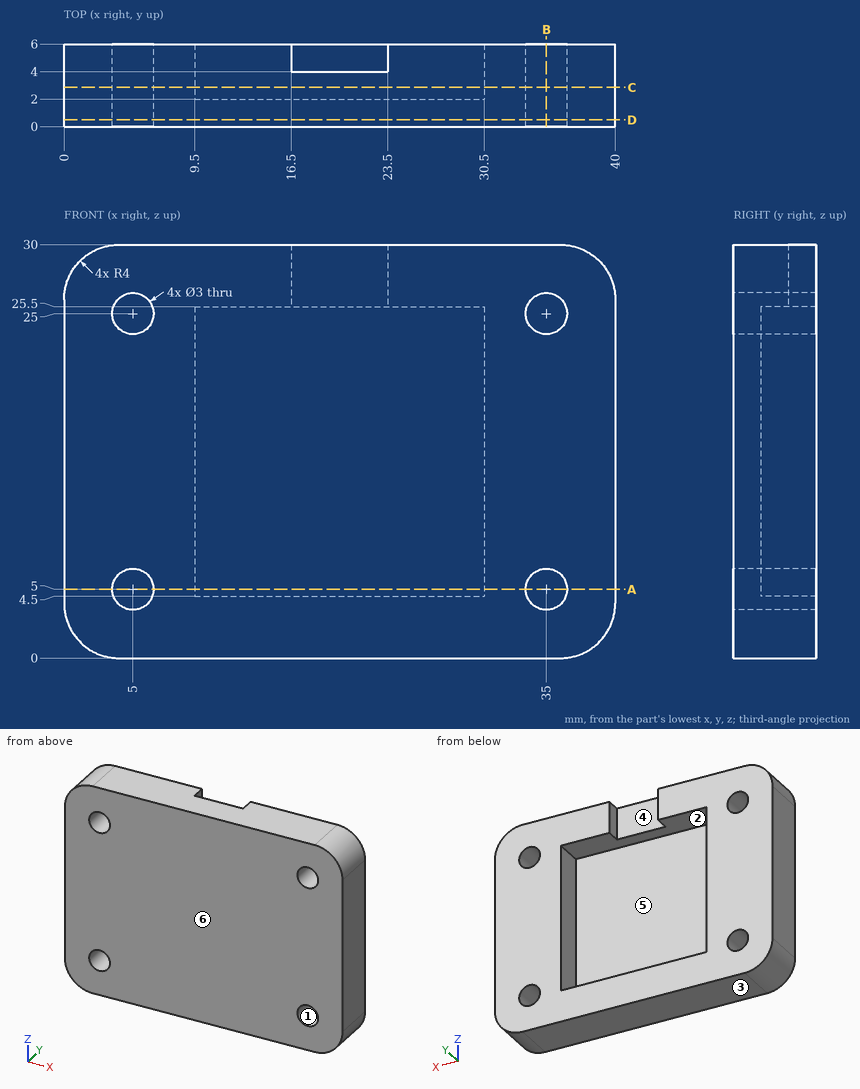
Drawing for the job (mm, zero at the part's lowest x, y, z). A direction names the side the tool comes from. Coordinates: 2 decimals unless noted, no trailing zeros. Loops run counter-clockwise (first coordinate to the right, second up) from the corner with the lowest first, then second, coordinate; pieces in that order, holes last. Notation, with made-up numbers: (68.5, -10) - (115.5, -10) arc R15 ccw to (115.5, 14) - close; hole circle Ø9 at (-21, -30.5). An arc over 180 degrees is marked (long way). Return JSON: item names as keys, results as strings.
1. Drop flat-ended pins along their axis: pin 1 (3.5 mm diameter, centred on x = 19, z = 26.5, fed in from +Y); pin 2 (6.5 mm diameter, centred on x = 18.5, z = 14.5, fed in from +Y); pin 3 (0.6 mm diameter, centred on y = 5.5, z = 27, fed in from +X). Give the stop position or say it passes through.
Result:
{"pin 1": "stops at y = 4", "pin 2": "stops at y = 2", "pin 3": "stops at x = 39.94"}
2. Band-saw the part on C-C (y = 2.85). Give the cut face in (x, z), and give its area (3 significant figures).
Result:
{"outline": "(0, 4) arc R4 ccw to (4, 0) - (36, 0) arc R4 ccw to (40, 4) - (40, 26) arc R4 ccw to (36, 30) - (4, 30) arc R4 ccw to (0, 26) - close; hole circle Ø3 at (5, 5); hole circle Ø3 at (5, 25); hole (9.5, 4.5) - (30.5, 4.5) - (30.5, 25.5) - (9.5, 25.5) - close; hole circle Ø3 at (35, 5); hole circle Ø3 at (35, 25)", "area": "717 mm2"}
3. Band-saw the part on D-D (y = 0.5). Give the cut face in (x, z), and give its area (3 significant figures).
Result:
{"outline": "(0, 4) arc R4 ccw to (4, 0) - (36, 0) arc R4 ccw to (40, 4) - (40, 26) arc R4 ccw to (36, 30) - (4, 30) arc R4 ccw to (0, 26) - close; hole circle Ø3 at (5, 5); hole circle Ø3 at (5, 25); hole circle Ø3 at (35, 5); hole circle Ø3 at (35, 25)", "area": "1,160 mm2"}
4. Band-saw the part on A-A (z = 5). Give the cut face in (x, y), and give its area (3 significant figures).
Result:
{"outline": "(0, 0) - (3.5, 0) - (3.5, 6) - (0, 6) - close; (6.5, 0) - (33.5, 0) - (33.5, 6) - (30.5, 6) - (30.5, 2) - (9.5, 2) - (9.5, 6) - (6.5, 6) - close; (36.5, 0) - (40, 0) - (40, 6) - (36.5, 6) - close", "area": "120 mm2"}
5. 3-axis set-ups, long thin cutter, end or side, ignore diameter. For the marked faces 5 and 6: which of +Z, -Z, +X, -X, +Y, -Y reach the whole face in a straight line?
Result:
{"face 5": "+Y", "face 6": "+Z, -Z, +X, -X, -Y"}
6. Probe L1, parallel to X at y = 1.2, z = 25; L2, parallel to X at y = 2.2, z = 25; L3, parallel to Z at x = 25, y = 4.95. List the from-to ranges inside material, lowest first. Write a range as from..to.
Result:
{"L1": "x = 0..3.5, 6.5..33.5, 36.5..40", "L2": "x = 0..3.5, 6.5..9.5, 30.5..33.5, 36.5..40", "L3": "z = 0..4.5, 25.5..30"}
7. Mould opens along Z. For the marked faces 1, 2, 3 and 4 say: released by +Z, released by -Z, zero draft, split by the parting line, or undercut.
Result:
{"face 1": "undercut", "face 2": "undercut", "face 3": "released by -Z", "face 4": "zero draft"}
8. Band-saw the part on B-B (x = 35). Give the cut face in (y, z), and give its area (3 significant figures).
Result:
{"outline": "(0, 0) - (6, 0) - (6, 3.5) - (0, 3.5) - close; (0, 6.5) - (6, 6.5) - (6, 23.5) - (0, 23.5) - close; (0, 26.5) - (6, 26.5) - (6, 30) - (0, 30) - close", "area": "144 mm2"}
